```python
from build123d import *

# Parameters (mm, degrees)
SKETCH1_R           = 6.35
BOSS_EXTRUDE1_DEPTH = 6.35
SKETCH3_R           = 9.525
BOSS_EXTRUDE2_DEPTH = 3.175
SKETCH4_W           = 9.652
SKETCH4_H           = 6.35
CUT_EXTRUDE2_DEPTH  = 17.497783942


with BuildPart() as part:
    # Sketch1 → Boss-Extrude1 (new body)
    with BuildSketch(Plane.XY):
        Circle(SKETCH1_R)
    extrude(amount=BOSS_EXTRUDE1_DEPTH)

    # Sketch3 → Boss-Extrude2 (add)
    with BuildSketch(Plane(origin=(0, 0, 0), x_dir=(-1, 0, 0), z_dir=(0, 0, -1))):
        Circle(SKETCH3_R)
    extrude(amount=BOSS_EXTRUDE2_DEPTH)

    # Sketch4 → Cut-Extrude2 (cut, through all)
    with BuildSketch(Plane(origin=(0, 0, -3.175), x_dir=(-1, 0, 0), z_dir=(0, 0, -1))):
        Rectangle(SKETCH4_W, SKETCH4_H)
    extrude(amount=-CUT_EXTRUDE2_DEPTH, mode=Mode.SUBTRACT)


solid = part.part
```
Model file for the job. Use its own axes, mm. A direction names the side the tool comes from. Give positions to 0.01 mm unless a question says otherwise; leave off trailing zeros. Write each loop counter-clockwise with the first axis right and the second up, starting at its lowest first coordinate (ties: lowest second). Pieces come first, ordered by that corner, then holes. Notation, with made-up numbers: (22.5, 66.25) -> (63.5, 66.25) arc R10 cw to (63.5, 84.25) -> close; hole circle Ø3 at (-13.75, -10.5). An arc over 180 degrees is marked (long way). Use CSV: the item, a comma, the result in double quotes. Start each with the question number.
1) Pin check, flat tips, straight feed: P1, Ø3, axis at y = 7.5, z = 0.5, coming from the +X side; P2, Ø1.5, axis at y = 3.5, z = 5, coming from the +X side; P3, Ø1, axis at y = -2, z = 2, coming from the -X side. Stop position of each tip, or through.
2) Tool access for faces 1 (the flat face through (0, -4, 6.35)), 2 (the flat face through (4.826, 0, 2)), 3 (the cylindrical face through (-1.38, -6.2, 3.13)): list every direction of +Z, -Z, +X, -X, +Y, -Y with a clear straight run to the whole face (end or side of a thin tool).
3) Cut at D-D on y = 4. List the corners of the cut face in (x, z) (3 decimals).
4) Drill centre lines: L1, parallel to Y at x = 0, z = 4.75 (3 decimals); L2, parallel to Z at x = 8, y = 2.25 (3 decimals); L3, parallel to Y at x = -3.75, z = 1.25 (3 decimals). Where is each one in solid material? Low to high.
5) Cut at B-B on y = 0. List the corners of the cut face in (x, z) (3 decimals).
6) Two-plate mould, pull along X, no slides. Class faces 4 (the cylindrical face through (7.559, -5.796, -1.565)), 5 (the flat face through (0, -4, -3.175)), 6 (the flat face through (0, -3.175, 2)): released by +X, released by -X, zero draft, split by the parting line, or undercut.
7) Cut at C-C on z = -1. List the corners of the cut face in (x, y) (3 decimals).
8) Cut at A-A on x = 0. List the corners of the cut face in (y, z) (3 decimals), plus the area to 3 significant figures.
Final values:
1,P1,"stops at x = 7.33"
1,P2,"stops at x = 5.72"
1,P3,"stops at x = -6.17"
2,face 1,"+Z, +X, -X, +Y, -Y"
2,face 2,"+Z, -Z"
2,face 3,"+Z"
3,outline,"(-8.644, -3.175) -> (8.644, -3.175) -> (8.644, 0) -> (4.932, 0) -> (4.932, 6.35) -> (-4.932, 6.35) -> (-4.932, 0) -> (-8.644, 0) -> close"
4,L1,"y = -6.35 to -3.175, 3.175 to 6.35"
4,L2,"z = -3.175 to 0"
4,L3,"y = -5.124 to -3.175, 3.175 to 5.124"
5,outline,"(-9.525, -3.175) -> (-4.826, -3.175) -> (-4.826, 6.35) -> (-6.35, 6.35) -> (-6.35, 0) -> (-9.525, 0) -> close; (4.826, -3.175) -> (9.525, -3.175) -> (9.525, 0) -> (6.35, 0) -> (6.35, 6.35) -> (4.826, 6.35) -> close"
6,face 4,"split by the parting line"
6,face 5,"zero draft"
6,face 6,"undercut"
7,outline,"circle Ø19.05 at (0, 0); hole (-4.826, -3.175) -> (4.826, -3.175) -> (4.826, 3.175) -> (-4.826, 3.175) -> close"
8,outline,"(-9.525, -3.175) -> (-3.175, -3.175) -> (-3.175, 6.35) -> (-6.35, 6.35) -> (-6.35, 0) -> (-9.525, 0) -> close; (3.175, -3.175) -> (9.525, -3.175) -> (9.525, 0) -> (6.35, 0) -> (6.35, 6.35) -> (3.175, 6.35) -> close"
8,area,"80.6 mm2"
